Autodesk Inventor part; units mm, degrees
ref_plane "YZ Plane" through (0, 0, 0) normal (1, 0, 0) x (0, 1, 0)
ref_plane "XZ Plane" through (0, 0, 0) normal (0, 1, 0) x (-1, 0, 0)
ref_plane "XY Plane" through (0, 0, 0) normal (0, 0, 1) x (1, 0, 0)
sketch "Sketch5" plane through (0, 0, 0) normal (0, 0, 1) x (1, 0, 0)
  line L0 (0, -500) -> (900, -500)
  line L1 (900, -500) -> (900, 850)
  line L2 (900, 850) -> (0, 850)
  line L3 (0, 850) -> (0, -500)
  line L4 (0, -500) -> (900, 850) construction
  line L5 (900, -500) -> (0, 850) construction
  line L6 (300, 700) -> (600, 700)
  line L7 (750, 550) -> (750, -200)
  line L8 (600, -350) -> (300, -350)
  line L9 (150, -200) -> (150, 550)
  arc A0 (750, 550) -> (600, 700) centre (600, 550) ccw
  arc A1 (300, 700) -> (150, 550) centre (300, 550) ccw
  arc A2 (150, -200) -> (300, -350) centre (300, -200) ccw
  arc A3 (600, -350) -> (750, -200) centre (600, -200) ccw
  line L10 (600, 697) -> (300, 697)
  arc A4 (300, 697) -> (153, 550) centre (300, 550) ccw
  line L11 (153, 550) -> (153, -200)
  arc A5 (153, -200) -> (300, -347) centre (300, -200) ccw
  line L12 (300, -347) -> (600, -347)
  arc A6 (600, -347) -> (747, -200) centre (600, -200) ccw
  line L13 (747, -200) -> (747, 550)
  arc A7 (747, 550) -> (600, 697) centre (600, 550) ccw
  point P0 (0, 0)
  point P1 (450, 175)
  dimension "d0" = 900
  dimension "d1" = 1350
  dimension "d2" = 150
  dimension "d3" = 150
  dimension "d4" = 150
  dimension "d5" = 150
  dimension "d6" = 150
  dimension "d9" = 3
extrude "Extrusion1" add sketch "Sketch5" along normal mid plane 3.048 contours L6 A0 L7 A3 L8 A2 L9 A1
sketch "Sketch6" plane through (0, 0, 1.524) normal (0, 0, 1) x (1, 0, 0)
  line L0 (300, -350) -> (600, -350)
  arc A0 (600, -350) -> (750, -200) centre (600, -200) ccw
  line L1 (750, -200) -> (750, 550)
  arc A1 (750, 550) -> (600, 700) centre (600, 550) ccw
  line L2 (600, 700) -> (300, 700)
  arc A2 (300, 700) -> (150, 550) centre (300, 550) ccw
  line L3 (150, 550) -> (150, -200)
  arc A3 (150, -200) -> (300, -350) centre (300, -200) ccw
  arc A4 (747, 550) -> (600, 697) centre (600, 550) ccw
  line L4 (747, 550) -> (747, -200)
  arc A5 (600, -347) -> (747, -200) centre (600, -200) ccw
  line L5 (600, -347) -> (300, -347)
  arc A6 (153, -200) -> (300, -347) centre (300, -200) ccw
  line L6 (153, -200) -> (153, 550)
  arc A7 (300, 697) -> (153, 550) centre (300, 550) ccw
  line L7 (300, 697) -> (600, 697)
  line L8 (300, 708) -> (600, 708)
  arc A8 (758, 550) -> (600, 708) centre (600, 550) ccw
  line L9 (758, 550) -> (758, -200)
  arc A9 (600, -358) -> (758, -200) centre (600, -200) ccw
  line L10 (600, -358) -> (300, -358)
  arc A10 (142, -200) -> (300, -358) centre (300, -200) ccw
  line L11 (142, -200) -> (142, 550)
  arc A11 (300, 708) -> (142, 550) centre (300, 550) ccw
  arc A12 (741, 550) -> (600, 691) centre (600, 550) ccw
  line L12 (741, 550) -> (741, -200)
  arc A13 (600, -341) -> (741, -200) centre (600, -200) ccw
  line L13 (600, -341) -> (300, -341)
  arc A14 (159, -200) -> (300, -341) centre (300, -200) ccw
  line L14 (159, -200) -> (159, 550)
  arc A15 (300, 691) -> (159, 550) centre (300, 550) ccw
  line L15 (300, 691) -> (600, 691)
  point P0 (0, 0)
  dimension "d12" = 8
  dimension "d13" = 6
extrude "Extrusion2" add sketch "Sketch6" along normal blind 4 contours A3 L3 A2 L2 A1 L1 A0 L0 | L4 A5 L5 A6 L6 A7 L7 A4 | L8 A8 L9 A9 L10 A10 L11 A11
sketch "Sketch7" plane through (0, 0, -1.524) normal (0, 0, -1) x (-1, 0, 0)
  line L0 (-300, -358) -> (-600, -358)
  arc A0 (-300, -358) -> (-142, -200) centre (-300, -200) ccw
  line L1 (-142, 550) -> (-142, -200)
  arc A1 (-142, 550) -> (-300, 708) centre (-300, 550) ccw
  line L2 (-600, 708) -> (-300, 708)
  arc A2 (-600, 708) -> (-758, 550) centre (-600, 550) ccw
  line L3 (-758, -200) -> (-758, 550)
  arc A3 (-758, -200) -> (-600, -358) centre (-600, -200) ccw
  arc A4 (-300, -350) -> (-150, -200) centre (-300, -200) ccw
  line L4 (-300, -350) -> (-600, -350)
  arc A5 (-750, -200) -> (-600, -350) centre (-600, -200) ccw
  line L5 (-750, -200) -> (-750, 550)
  arc A6 (-600, 700) -> (-750, 550) centre (-600, 550) ccw
  line L6 (-600, 700) -> (-300, 700)
  arc A7 (-150, 550) -> (-300, 700) centre (-300, 550) ccw
  line L7 (-150, 550) -> (-150, -200)
  line L8 (-600, -350) -> (-300, -350)
  arc A8 (-300, -350) -> (-150, -200) centre (-300, -200) ccw
  line L9 (-150, -200) -> (-150, 550)
  arc A9 (-150, 550) -> (-300, 700) centre (-300, 550) ccw
  line L10 (-300, 700) -> (-600, 700)
  arc A10 (-600, 700) -> (-750, 550) centre (-600, 550) ccw
  line L11 (-750, 550) -> (-750, -200)
  arc A11 (-750, -200) -> (-600, -350) centre (-600, -200) ccw
  arc A12 (-600, 697) -> (-747, 550) centre (-600, 550) ccw
  line L12 (-600, 697) -> (-300, 697)
  arc A13 (-153, 550) -> (-300, 697) centre (-300, 550) ccw
  line L13 (-153, 550) -> (-153, -200)
  arc A14 (-300, -347) -> (-153, -200) centre (-300, -200) ccw
  line L14 (-300, -347) -> (-600, -347)
  arc A15 (-747, -200) -> (-600, -347) centre (-600, -200) ccw
  line L15 (-747, -200) -> (-747, 550)
  line L16 (-600, -341) -> (-300, -341)
  arc A16 (-741, -200) -> (-600, -341) centre (-600, -200) ccw
  line L17 (-741, 550) -> (-741, -200)
  arc A17 (-600, 691) -> (-741, 550) centre (-600, 550) ccw
  line L18 (-300, 691) -> (-600, 691)
  arc A18 (-159, 550) -> (-300, 691) centre (-300, 550) ccw
  line L19 (-159, -200) -> (-159, 550)
  arc A19 (-300, -341) -> (-159, -200) centre (-300, -200) ccw
  line L20 (-300, 697) -> (-600, 697)
  arc A20 (-600, 697) -> (-747, 550) centre (-600, 550) ccw
  line L21 (-747, 550) -> (-747, -200)
  arc A21 (-747, -200) -> (-600, -347) centre (-600, -200) ccw
  line L22 (-600, -347) -> (-300, -347)
  arc A22 (-300, -347) -> (-153, -200) centre (-300, -200) ccw
  line L23 (-153, -200) -> (-153, 550)
  arc A23 (-153, 550) -> (-300, 697) centre (-300, 550) ccw
  point P0 (0, 0)
extrude "Extrusion3" add sketch "Sketch7" along normal blind 4 contours L0 A3 L3 A2 L2 A1 L1 A0 | L4 A5 L5 A6 L6 A7 L7 A4 | L12 A13 L13 A14 L14 A15 L15 A12
equation "\"d10\" = Thickness"
equation "\"BendRadius\" = Thickness"
equation "\"BendReliefWidth\" = Thickness"
equation "\"BendReliefDepth\" = 0.5 * Thickness"
equation "\"CornerReliefSize\" = 4 * Thickness"
equation "\"MinimumRemnant\" = 2 * Thickness"
equation "\"TransitionRadius\" = BendRadius"
equation "\"JacobiRadiusSize\" = BendRadius"
equation "\"GapSize\" = Thickness"
equation "\"Space5\" = 0"
equation "\"Space6\" = 0"
equation "\"Space7\" = 0"
properties part number "Caucho"
The listing builds one solid part. Answer for the finished solid, in the listing's coordinates (mm). A direction names the side the tool comes from. Give positions to 0.01 mm unless a question says otherwise; leave off trailing zeros. Loops run counter-clockwise (first coordinate to the right, second up) from the corner with the lowest first, then second, coordinate; pieces in that order, holes last. Notation, with made-up numbers: M 69,2 L 110,2 A11 cw 110,12 Z; hole C -13,82.5 d2. An arc over 180 degrees is marked long. One line per item, written item: value.
Q1. A cutting plane is placed at B-B on x = 425.5. Determine the outline of the cut face in (y, z), then the cut area to 3 significant figures.
Working result:
outline: M -358,-5.52 L -341,-5.52 L -341,-1.52 L -347,-1.52 L -347,1.52 L -341,1.52 L -341,5.52 L -358,5.52 L -358,1.52 L -350,1.52 L -350,-1.52 L -358,-1.52 Z; M 691,-5.52 L 708,-5.52 L 708,-1.52 L 700,-1.52 L 700,1.52 L 708,1.52 L 708,5.52 L 691,5.52 L 691,1.52 L 697,1.52 L 697,-1.52 L 691,-1.52 Z
area: 290 mm^2
Q2. Find the intervals of material crossed by line 1 (Y direction, x = 462, z = 2.25); line 2 (X direction, y = 198, z = -0.5); line 3 (X direction, y = -80.5, z = 2.5), in increasing order. Write a range as from..to.
Working result:
line 1: y = -358..-341, 691..708
line 2: x = 150..153, 747..750
line 3: x = 142..159, 741..758
Q3. Determine the mould class of faces 1 (the face through (705.081, -302.796, -0.021)), 2 (the face through (189.51, 662.94, -3.5)), 3 (the face through (698.6, 650.79, 3.5)), 4 (the face through (710.49, -312.94, -3.5)) for opening direction Y: +Y half, -Y half, draft (parallel to the pull), parting line (faces both ways), or undercut.
Working result:
face 1: undercut
face 2: +Y half
face 3: undercut
face 4: -Y half
Q4. For faces 5 (the face through (201.4, 650.79, -3.5)), 6 (the face through (197.204, -305.081, -0.021)), 7 (the face through (195.11, -307.23, -0.02)), 8 (the face through (704.89, 657.23, -0.02)), determine the directions among +Z, -Z, +X, -X, +Y, -Y from which every point of the face is accessible in a straight line to the end or side of a thin tool.
Working result:
face 5: +Z, -Z
face 6: none
face 7: -X, -Y
face 8: +X, +Y
Q5. A cutting plane is placed at A-A on y = 233. Determine the outline of the cut face in (x, z).
Working result:
outline: M 142,-5.52 L 159,-5.52 L 159,-1.52 L 153,-1.52 L 153,1.52 L 159,1.52 L 159,5.52 L 142,5.52 L 142,1.52 L 150,1.52 L 150,-1.52 L 142,-1.52 Z; M 741,-5.52 L 758,-5.52 L 758,-1.52 L 750,-1.52 L 750,1.52 L 758,1.52 L 758,5.52 L 741,5.52 L 741,1.52 L 747,1.52 L 747,-1.52 L 741,-1.52 Z
Q6. A cutting plane is placed at C-C on z = -3.25. Determine the outline of the cut face in (x, y), then the cut area to 3 significant figures.
Working result:
outline: M 142,-200 A158 ccw 300,-358 L 600,-358 A158 ccw 758,-200 L 758,550 A158 ccw 600,708 L 300,708 A158 ccw 142,550 Z; hole M 159,-200 A141 ccw 300,-341 L 600,-341 A141 ccw 741,-200 L 741,550 A141 ccw 600,691 L 300,691 A141 ccw 159,550 Z
area: 51,700 mm^2
Q7. Flat-ended cylindrical pins translate along their axes: P1, Ø1.5, axis at x = 513.5, z = -0.5, coming from the -Y side; P2, Ø5, axis at x = 210, z = -3.5, coming from the -Y side; P3, Ø1, axis at x = 296.5, z = -1.5, coming from the -Y side. Find the tip coordinate at first contact, or state that the pin passes through.
Working result:
P1: stops at y = -350
P2: stops at y = -331.56
P3: stops at y = -357.97
